Verification items for the finished model (mm, model axes). A direction names the side the tool comes from. Round coordinates to 2 decimals unless told otherwise and drop trailing zeros. Write each loop counter-clockwise with the first axis right and the second up, starting at its lowest first coordinate (ties: lowest second). Pieces come first, ordered by that corner, then holes.
from build123d import *

# Parameters (mm, degrees)
AUFSATZ_LINEAR_AUSTRAGEN1_DEPTH = 3
SKIZZE2_R                       = 1.7
SCHNITT_LINEAR_AUSTRAGEN1_DEPTH = 4
DURCHGANGSLOCH_F_R_M41_D        = 4.5
DURCHGANGSLOCH_F_R_M31_D        = 3.4
VERRUNDUNG1_R                   = 2


with BuildPart() as part:
    # Skizze1 → Aufsatz-Linear austragen1 (new body)
    with BuildSketch(Plane.XY):
        with BuildLine():
            Line((0, 0), (0, -9))
            Line((0, -9), (-5, -9))
            Line((-5, -9), (-5, -21))
            ThreePointArc((-5, -21), (-10, -26), (-15, -21))
            Line((-15, -21), (-15, -9))
            Line((-15, -9), (-20, -9))
            Line((-20, -9), (-20, 20))
            Line((-20, 20), (50, 20))
            Line((50, 20), (50, 0))
            Line((50, 0), (0, 0))
        make_face()
    extrude(amount=AUFSATZ_LINEAR_AUSTRAGEN1_DEPTH)

    # Skizze2 → Schnitt-Linear austragen1 (cut, through all)
    with BuildSketch(Plane.XY.offset(3)):
        with Locations((-10, -21)):
            Circle(SKIZZE2_R)
    extrude(amount=-SCHNITT_LINEAR_AUSTRAGEN1_DEPTH, mode=Mode.SUBTRACT)

    # Durchgangsloch für M41 (through all)
    with Locations(Plane.XY.offset(3)):
        with Locations((20, 10), (40, 10)):
            Hole(DURCHGANGSLOCH_F_R_M41_D / 2)

    # Durchgangsloch für M31 (through all)
    with Locations(Plane.XY.offset(3)):
        with Locations((-17.5, 12), (-2.5, -4), (-17.5, -4)):
            Hole(DURCHGANGSLOCH_F_R_M31_D / 2)

    # Verrundung1
    verrundung1_edges = [part.edges().sort_by_distance(p)[0] for p in [
        (0, 0, 1.5),
        (0, -9, 1.5),
        (-5, -9, 1.5),
        (-15, -9, 1.5),
        (-20, -9, 1.5),
        (-20, 20, 1.5),
        (50, 20, 1.5),
        (50, 0, 1.5),
    ]]
    fillet(verrundung1_edges, radius=VERRUNDUNG1_R)


solid = part.part
Q1. Sectioned sample at C-C (y = 11). Enter the section's corners in (x, z).
Recorded:
outline: (-20, 0) - (-18.87, 0) - (-18.87, 3) - (-20, 3) - close; (-16.13, 0) - (17.98, 0) - (17.98, 3) - (-16.13, 3) - close; (22.02, 0) - (37.98, 0) - (37.98, 3) - (22.02, 3) - close; (42.02, 0) - (50, 0) - (50, 3) - (42.02, 3) - close
Q2. Sectioned sample at A-A (x = -10). Enter the section's corners in (y, z), plus the area to 3 significant figures.
Recorded:
outline: (-26, 0) - (-22.7, 0) - (-22.7, 3) - (-26, 3) - close; (-19.3, 0) - (20, 0) - (20, 3) - (-19.3, 3) - close
area: 128 mm2
Q3. Release check for a two-part mould opening along X. For faces 3 (the cylindrical face through (-4.4, -9.57, 1.52)), 4 (the cylindrical face through (42.248, 10.099, 1.479)), 5 (the flat face through (15, 20, 1)) record: released by +X, released by -X, zero draft, split by the parting line, or undercut.
Recorded:
face 3: released by +X
face 4: undercut
face 5: zero draft
Q4. Material ranges on line 1 along Y through (x, z) = (40, 1.75); line 2 along Y through (x, z) = (-10, 1.3); line 3 along Y through (x, z) = (33, 1.55), recorded low to high.
Recorded:
line 1: y = 0 to 7.75, 12.25 to 20
line 2: y = -26 to -22.7, -19.3 to 20
line 3: y = 0 to 20
Q5. Depth check by flat-ended pin: P1, Ø0.5, axis at x = -2.5, z = 1, coming from the -Y side; P2, Ø1.5, axis at y = -18, z = 1, coming from the -X side; P3, Ø1.5, axis at y = -5, z = 1, coming from the +X side. Enter the tip coordinate at first touch or a pass-through.
Recorded:
P1: stops at y = -9
P2: stops at x = -15
P3: stops at x = 0
Q6. Tool access check on faces 1 (the cylindrical face through (-9.086, -19.567, 1.521)), 2 (the flat face through (0, -4, 1)). Record the directions out of +Z, -Z, +X, -X, +Y, -Y that give a thin tool (end or side, any length) a straight path to the whole face; none if there is none.
Recorded:
face 1: +Z, -Z
face 2: +Z, -Z, +X, -Y
Q7. Sectioned sample at D-D (x = 40). Enter the section's corners in (y, z), plus the area to 3 significant figures.
Recorded:
outline: (0, 0) - (7.75, 0) - (7.75, 3) - (0, 3) - close; (12.25, 0) - (20, 0) - (20, 3) - (12.25, 3) - close
area: 46.5 mm2
Q8. Sectioned sample at B-B (z = 1.25). Enter the section's corners in (x, y).
Recorded:
outline: (-20, -7) arc R2 ccw to (-18, -9) - (-17, -9) arc R2 cw to (-15, -11) - (-15, -21) arc R5 ccw to (-5, -21) - (-5, -11) arc R2 cw to (-3, -9) - (-2, -9) arc R2 ccw to (0, -7) - (0, -2) arc R2 cw to (2, 0) - (48, 0) arc R2 ccw to (50, 2) - (50, 18) arc R2 ccw to (48, 20) - (-18, 20) arc R2 ccw to (-20, 18) - close; hole circle Ø3.4 at (-17.5, -4); hole circle Ø3.4 at (-17.5, 12); hole circle Ø3.4 at (-10, -21); hole circle Ø3.4 at (-2.5, -4); hole circle Ø4.5 at (20, 10); hole circle Ø4.5 at (40, 10)
